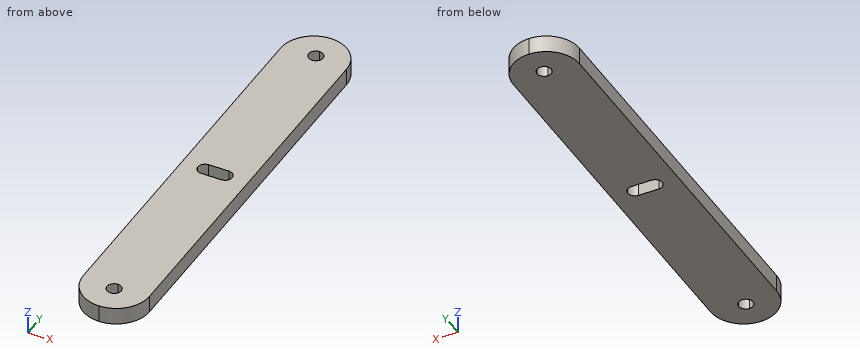
from build123d import *

# Parameters (mm, degrees)
F1_DEPTH = 3


with BuildPart() as f1:
    # F0 (on Top) → F1 (new body)
    with BuildSketch(Plane.XY):
        with BuildLine():
            Line((1.154214, 32.75), (1.154214, 0))
            Line((1.154214, 0), (3.904214, 0))
            ThreePointArc((3.904214, 0), (4.27033, 0.883883), (5.154214, 1.25))
            Line((5.154214, 1.25), (6.904214, 1.25))
            Line((6.904214, 1.25), (6.904214, 32.252756))
            ThreePointArc((6.904214, 32.252756), (5.65697, 33.5), (6.904214, 34.747244))
            Line((6.904214, 34.747244), (6.904214, 38.5))
            ThreePointArc((6.904214, 38.5), (2.83835, 36.815864), (1.154214, 32.75))
        make_face()
        with BuildLine():
            Line((3.904214, 0), (1.154214, 0))
            Line((1.154214, 0), (1.154214, -32.75))
            ThreePointArc((1.154214, -32.75), (2.83835, -36.815864), (6.904214, -38.5))
            Line((6.904214, -38.5), (6.904214, -34.747244))
            ThreePointArc((6.904214, -34.747244), (5.65697, -33.5), (6.904214, -32.252756))
            Line((6.904214, -32.252756), (6.904214, -1.25))
            Line((6.904214, -1.25), (5.154214, -1.25))
            ThreePointArc((5.154214, -1.25), (4.27033, -0.883883), (3.904214, 0))
        make_face()
        with BuildLine():
            ThreePointArc((12.654214, 32.75), (10.970078, 36.815864), (6.904214, 38.5))
            Line((6.904214, 38.5), (6.904214, 34.747244))
            ThreePointArc((6.904214, 34.747244), (7.786148, 34.381934), (8.151457, 33.5))
            ThreePointArc((8.151457, 33.5), (7.786148, 32.618066), (6.904214, 32.252756))
            Line((6.904214, 32.252756), (6.904214, 1.25))
            Line((6.904214, 1.25), (8.654214, 1.25))
            ThreePointArc((8.654214, 1.25), (9.538097, 0.883883), (9.904214, 0))
            Line((9.904214, 0), (12.654214, 0))
            Line((12.654214, 0), (12.654214, 32.75))
        make_face()
        with BuildLine():
            Line((6.904214, -34.747244), (6.904214, -38.5))
            ThreePointArc((6.904214, -38.5), (10.970078, -36.815864), (12.654214, -32.75))
            Line((12.654214, -32.75), (12.654214, 0))
            Line((12.654214, 0), (9.904214, 0))
            ThreePointArc((9.904214, 0), (9.538097, -0.883883), (8.654214, -1.25))
            Line((8.654214, -1.25), (6.904214, -1.25))
            Line((6.904214, -1.25), (6.904214, -32.252756))
            ThreePointArc((6.904214, -32.252756), (7.786148, -32.618066), (8.151457, -33.5))
            ThreePointArc((8.151457, -33.5), (7.786148, -34.381934), (6.904214, -34.747244))
        make_face()
    extrude(amount=F1_DEPTH)


solid = f1.part
Check sheet for the modelled part. Datum: model origin and axes. Units: mm. Give positions to 0.01 mm unless a question says otherwise; leave off trailing zeros. Write each loop counter-clockwise with the first axis right and the second up, starting at its lowest first coordinate (ties: lowest second). Pieces come first, ordered by that corner, then holes. Notation, with made-up numbers: M 58.5,20.25 L 82.5,20.25 A29 ccw 82.5,49.25 Z; hole C -19.5,74.5 d7. An arc over 180 degrees is marked long. Use one line per item in the form item = value.
(1) Material ranges on line 1 along Y through (x, z) = (6.75, 1.7); line 2 along Y through (x, z) = (9.5, 2.8); line 3 along X through (y, z) = (-34.5, 1.6), recorded low to high.
Answer block:
line_1 = -38.5 to -34.74, -32.26 to -1.25, 1.25 to 32.26, 34.74 to 38.5
line_2 = -37.88 to -0.92, 0.92 to 37.88
line_3 = 1.43 to 6.16, 7.65 to 12.38
(2) Section check B-B on x = 11.75. Record the boundary of the cut face in (y, z).
Answer block:
outline = M -35.85,0 L 35.85,0 L 35.85,3 L -35.85,3 Z
(3) Section check C-C on x = 2. Record the boundary of the cut face in (y, z).
Answer block:
outline = M -35.75,0 L 35.75,0 L 35.75,3 L -35.75,3 Z
(4) Section check A-A on z = 1.8. Record the boundary of the cut face in (x, y), plus the area to 3 significant figures.
Answer block:
outline = M 1.15,-32.75 A5.75 ccw 12.65,-32.75 L 12.65,32.75 A5.75 ccw 1.15,32.75 Z; hole M 5.15,-1.25 L 8.65,-1.25 A1.25 ccw 9.9,0 A1.25 ccw 8.65,1.25 L 5.15,1.25 A1.25 ccw Z; hole M 6.9,-34.75 A1.25 ccw 8.15,-33.5 A1.25 ccw 6.9,-32.25 A1.25 ccw Z; hole M 6.9,32.25 A1.25 ccw 8.15,33.5 A1.25 ccw 6.9,34.75 A1.25 ccw Z
area = 834 mm2
